Input: part model. Units: mm. Frame: model coordinates. Face numbers are marked on the shaded views. A direction names the side the tool comes from. Give positions to 0.01 mm unless a question says otherwise; leave off trailing zeros. Loops run counter-clockwise (first coordinate to the right, second up) from the corner with the lowest first, then second, coordinate; pieces in that order, holes last. Notation, with made-up numbers: M -39,66.5 L 19,66.5 A12 ccw 19,70.5 Z; hole C 55.5,71.5 d7. An arc over 180 degrees is marked long. Use CSV: the item, a comma, the result in double quotes. Start each with the question number.
Q1. Reachability of the marked faces 4 and 5 from +Z, -Z, +X, -X, +Y, -Y: full face, straight path, thin tool, end or side. Return the list, or none.
Q2. Material intervals for line 1 along Y through (x, z) = (43, -28) (3 decimals); line 2 along Z through (x, y) = (38.5, -10); line 3 along X through (y, z) = (-20, 4.5), sorted ascending.
Q3. Section D-D, the plane z = 40. Output: boundary loops of the cut face in (x, y) (3 decimals).
Q4. Pin query (flat end, axial travel): pin 1 (20.5 mm diameter, centred on y = -18.5, z = 5.5, fed in from -X); pin 2 (3.5 mm diameter, centred on x = -27.5, y = -40, fed in from -Z); pin 3 (12 mm diameter, centred on x = -11, z = 1, fed in from +Y) (3 decimals); pin 4 (5 mm diameter, centred on y = -28.5, z = 19, fed in from -X). Return the tip coordinate at first contact, or that it passes through.
Q5. Pull-direction query (Y, two-part tool) for the marked faces 1, 2 and 3; classes: released by +Y, released by -Y, zero draft, split by the parting line, or undercut.
Q6. Section C-C, the plane y = -24.5. Output: boundary loops of the cut face in (x, z).
Q7. Section B-B, the plane x = 42. Output: boundary loops of the cut face in (y, z) (3 decimals), plus the area to 3 significant figures.
Q8. Section A-A, the plane z = -3. Output: boundary loops of the cut face in (x, y) (3 decimals).
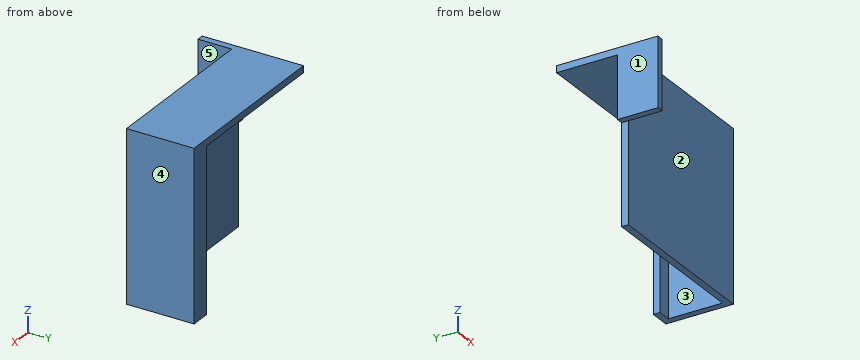
from build123d import *

# Parameters (mm, degrees)
F0_W      = 82.55
F0_H      = 76.2
F1_DEPTH  = 31.75
F2_W      = 79.375
F2_H      = 28.575
F3_DEPTH  = 101.6
F4_W      = 9.525
F4_H      = 76.2
F5_DEPTH  = 3.175
F7_DEPTH  = 3.175
F8_W      = 19.05
F8_H      = 79.375
F9_DEPTH  = 3.175
F10_W     = 19.05
F10_H     = 46.99
F11_DEPTH = 3.175


with BuildPart() as f1:
    # F0 (on Front) → F1 (new body)
    with BuildSketch(Plane.XZ):
        with Locations((12.593148, 4.577052)):
            Rectangle(F0_W, F0_H)
    extrude(amount=F1_DEPTH)

    # F2 (on face) → F3 (cut)
    with BuildSketch(Plane.XY.offset(42.677052)):
        with Locations((11.005648, -14.2875)):
            Rectangle(F2_W, F2_H)
    extrude(amount=-F3_DEPTH, mode=Mode.SUBTRACT)

    # F4 (on face) → F5 (join)
    with BuildSketch(Plane(origin=(0, 0, 0), x_dir=(-1, 0, 0), z_dir=(0, 1, 0))):
        with Locations((-49.105648, 4.577052)):
            Rectangle(F4_W, F4_H)
    extrude(amount=-F5_DEPTH)

    # F6 (on face) → F7 (join)
    with BuildSketch(Plane.XY.offset(42.677052)):
        Polygon((-28.681852, -31.75), (53.868148, -31.75), (53.868148, 0), (-28.681852, 0), (-28.681852, -28.575), align=None)
    extrude(amount=F7_DEPTH)

    # F8 (on face) → F9 (join)
    with BuildSketch(Plane(origin=(-28.681852, 0, 0), x_dir=(0, -1, 0), z_dir=(-1, 0, 0))):
        with Locations((38.1, 6.164552)):
            Rectangle(F8_W, F8_H)
    extrude(amount=-F9_DEPTH)

    # F10 (on face) → F11 (cut)
    with BuildSketch(Plane(origin=(-28.681852, 0, 0), x_dir=(0, -1, 0), z_dir=(-1, 0, 0))):
        with Locations((38.1, -10.027948)):
            Rectangle(F10_W, F10_H)
    extrude(amount=-F11_DEPTH, mode=Mode.SUBTRACT)


solid = f1.part
A:
1,face 4,"+Z, -Z, +X, +Y, -Y"
1,face 5,"+Z, -Z, +X, -Y"
2,line 1,"-31.75 to -28.575"
2,line 2,"42.68 to 45.85"
2,line 3,"50.69 to 53.87"
3,outline,"M -28.682,-47.625 L -25.507,-47.625 L -25.507,-31.75 L 53.868,-31.75 L 53.868,0 L 44.343,0 L 44.343,-3.175 L 50.693,-3.175 L 50.693,-28.575 L -28.682,-28.575 Z"
4,pin 1,"x = -25.51"
4,pin 2,"z = 13.47"
4,pin 3,"y = -28.575"
4,pin 4,"x = -28.68"
5,face 1,"zero draft"
5,face 2,"released by -Y"
5,face 3,"undercut"
6,outline,"M -28.68,42.68 L 50.69,42.68 L 50.69,-33.52 L 53.87,-33.52 L 53.87,45.85 L -28.68,45.85 Z"
7,outline,"M -31.75,-33.523 L -28.575,-33.523 L -28.575,42.677 L 0,42.677 L 0,45.852 L -31.75,45.852 Z"
7,area,"343 mm^2"
8,outline,"M -25.507,-31.75 L 53.868,-31.75 L 53.868,0 L 44.343,0 L 44.343,-3.175 L 50.693,-3.175 L 50.693,-28.575 L -25.507,-28.575 Z"
